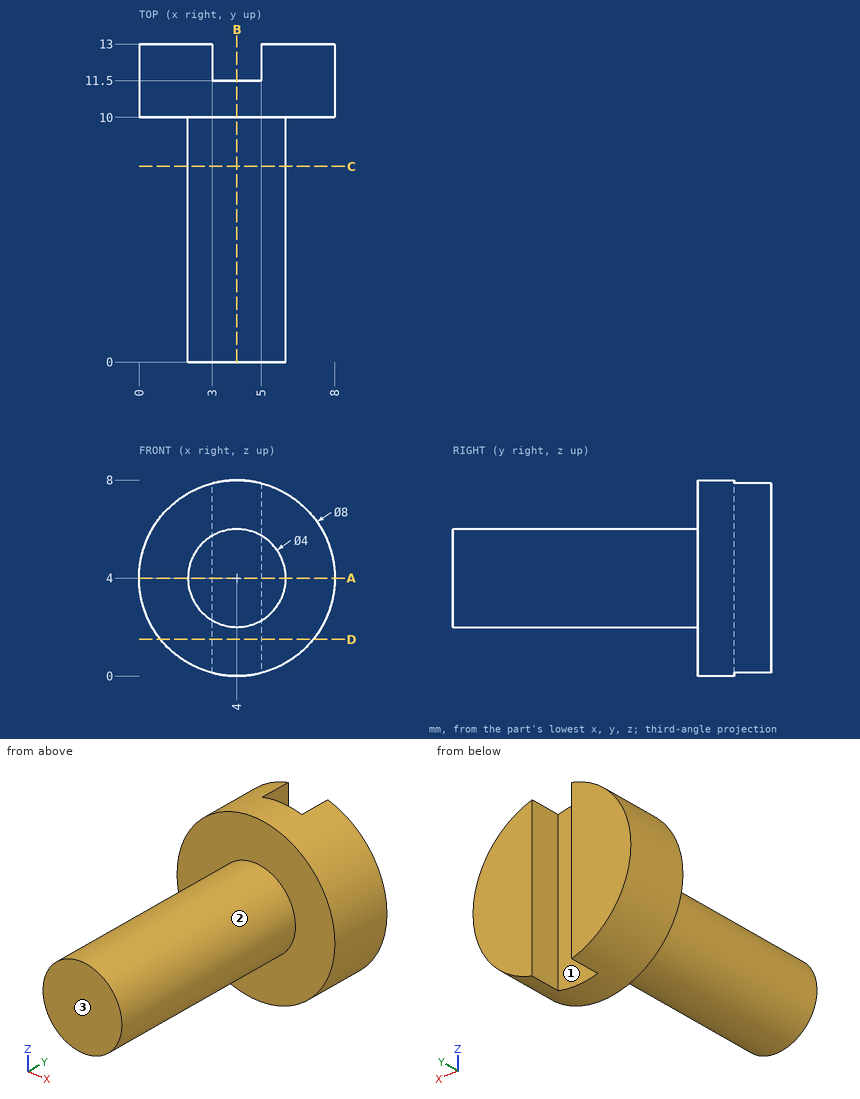
Geometry check sheet. Reference: drawing and pictorial views, mm from the part's lowest x, y, z. A direction names the side the tool comes from. Round coordinates to 2 decimals unless told otherwise and drop trailing zeros. Write each loop counter-clockwise with the first axis right and the second up, starting at its lowest first coordinate (ties: lowest second). Pieces come first, ordered by that corner, then holes. Notation, with made-up numbers: (-3, 54) -> (44, 54) arc R23 ccw to (44, 88) -> close; hole circle Ø1 at (-21, 1.25). An arc over 180 degrees is marked (long way). Answer as CSV lines item,"result". Start each with the question number.
1) Material ranges on line 1 (Y direction, x = 6.25, z = 6.25); line 2 (X direction, y = 8, z = 4); line 3 (X direction, y = 3.5, z = 2.75), recorded low to high. Write a range as from..to.
2) Section check C-C on y = 8. Enter the section's corners in (x, z).
3) Section check D-D on z = 1.5. Enter the section's corners in (x, y), and give its area (3 significant figures).
4) Section check B-B on x = 4. Enter the section's corners in (y, z), and give its area (3 significant figures).
5) Tool access check on the marked faces 1, 2 and 3. Record the directions out of +Z, -Z, +X, -X, +Y, -Y that give a thin tool (end or side, any length) a straight path to the whole face; none if there is none.
6) Go/stop test with flat-tipped pins: P1, Ø4, axis at x = 4.5, y = 3, coming from the -Z side; P2, Ø1.5, axis at x = 2.5, y = 2, coming from the +Z side; P3, Ø1, axis at x = 5, y = 11, coming from the -Z side. Record where each tip stops, or that it passes through.
7) Section check A-A on z = 4. Enter the section's corners in (x, y), and give its area (3 significant figures).
Found:
1,line 1,"y = 10..13"
1,line 2,"x = 2..6"
1,line 3,"x = 2.44..5.56"
2,outline,"circle Ø4 at (4, 4)"
3,outline,"(0.88, 10) -> (7.12, 10) -> (7.12, 13) -> (5, 13) -> (5, 11.5) -> (3, 11.5) -> (3, 13) -> (0.88, 13) -> close"
3,area,"15.7 mm^2"
4,outline,"(0, 2) -> (10, 2) -> (10, 0) -> (11.5, 0) -> (11.5, 8) -> (10, 8) -> (10, 6) -> (0, 6) -> close"
4,area,"52.0 mm^2"
5,face 1,"+Z, -Z, +Y"
5,face 2,"-Y"
5,face 3,"+Z, -Z, +X, -X, -Y"
6,P1,"stops at z = 2"
6,P2,"stops at z = 5.85"
6,P3,"stops at z = 0.03"
7,outline,"(0, 10) -> (2, 10) -> (2, 0) -> (6, 0) -> (6, 10) -> (8, 10) -> (8, 13) -> (5, 13) -> (5, 11.5) -> (3, 11.5) -> (3, 13) -> (0, 13) -> close"
7,area,"61.0 mm^2"
